from build123d import *
from OCP.BRepFilletAPI import BRepFilletAPI_MakeChamfer

# Parameters (mm, degrees)
BOSS_EXTRUDE1_DEPTH = 3
SKETCH2_R           = 2
CUT_EXTRUDE1_DEPTH  = 31.959580504
CHAMFER1_SIZE       = 2.38
CHAMFER1_SIZE2      = 1.109812226
SKETCH3_R           = 12.7
SKETCH3_R_2         = 11.375
BOSS_EXTRUDE2_DEPTH = 30.75
SKETCH5_W           = 5.58
SKETCH5_H           = 6.85
CUT_EXTRUDE3_DEPTH  = 10
CHAMFER3_SIZE       = 1
CHAMFER3_SIZE2      = 1.191753593
CUT_EXTRUDE4_START  = -5
SKETCH6_R           = 11.375
CUT_EXTRUDE4_DEPTH  = 5
CHAMFER4_SIZE       = 2.4293521
CHAMFER4_SIZE_2     = 3
FILLET1_R           = 0.5
CUT_EXTRUDE6_START  = -35
CUT_EXTRUDE6_DEPTH  = 35


with BuildPart() as part:
    # Sketch1 → Boss-Extrude1 (new body)
    with BuildSketch(Plane.XY):
        with BuildLine():
            Line((6.35, 28.075), (-6.35, 28.075))
            ThreePointArc((-6.35, 28.075), (-10.840128061, 26.215128061), (-12.7, 21.725))
            Line((-12.7, 21.725), (-12.7, -21.725))
            ThreePointArc((-12.7, -21.725), (-10.840128061, -26.215128061), (-6.35, -28.075))
            Line((-6.35, -28.075), (6.35, -28.075))
            ThreePointArc((6.35, -28.075), (10.840128061, -26.215128061), (12.7, -21.725))
            Line((12.7, -21.725), (12.7, 21.725))
            ThreePointArc((12.7, 21.725), (10.840128061, 26.215128061), (6.35, 28.075))
        make_face()
    extrude(amount=BOSS_EXTRUDE1_DEPTH)

    # Sketch2 → Cut-Extrude1 (cut, through all)
    with BuildSketch(Plane(origin=(0, 0, 0), x_dir=(-1, 0, 0), z_dir=(0, 0, -1))):
        with Locations((-7.7, -20.125)):
            Circle(SKETCH2_R)
        with Locations((-7.7, 20.125)):
            Circle(SKETCH2_R)
        with Locations((7.7, 20.125)):
            Circle(SKETCH2_R)
        with Locations((7.7, -20.125)):
            Circle(SKETCH2_R)
    extrude(amount=-CUT_EXTRUDE1_DEPTH, mode=Mode.SUBTRACT)

    # Chamfer1: one chamfer whose edges measure the first distance from different faces: ONE call of the kernel's chamfer builder (chamfer() names one face for all edges)
    chamfer1_edges_1 = [part.edges().sort_by_distance(p)[0] for p in [
        (-10.840128061, 26.215128061, 3),
    ]]
    chamfer1_side_1 = [part.faces().sort_by_distance(p)[0] for p in [
        (-10.840128061, 26.215128061, 1.5),
    ]]
    chamfer1_edges_2 = [part.edges().sort_by_distance(p)[0] for p in [
        (-12.7, 0, 3),
    ]]
    chamfer1_side_2 = [part.faces().sort_by_distance(p)[0] for p in [
        (-12.7, 0, 1.5),
    ]]
    chamfer1_edges_3 = [part.edges().sort_by_distance(p)[0] for p in [
        (-10.840128061, -26.215128061, 3),
    ]]
    chamfer1_side_3 = [part.faces().sort_by_distance(p)[0] for p in [
        (-10.840128061, -26.215128061, 1.5),
    ]]
    chamfer1_edges_4 = [part.edges().sort_by_distance(p)[0] for p in [
        (0, -28.075, 3),
    ]]
    chamfer1_side_4 = [part.faces().sort_by_distance(p)[0] for p in [
        (0, -28.075, 1.5),
    ]]
    chamfer1_edges_5 = [part.edges().sort_by_distance(p)[0] for p in [
        (10.840128061, -26.215128061, 3),
    ]]
    chamfer1_side_5 = [part.faces().sort_by_distance(p)[0] for p in [
        (10.840128061, -26.215128061, 1.5),
    ]]
    chamfer1_edges_6 = [part.edges().sort_by_distance(p)[0] for p in [
        (12.7, 0, 3),
    ]]
    chamfer1_side_6 = [part.faces().sort_by_distance(p)[0] for p in [
        (12.7, 0, 1.5),
    ]]
    chamfer1_edges_7 = [part.edges().sort_by_distance(p)[0] for p in [
        (10.840128061, 26.215128061, 3),
    ]]
    chamfer1_side_7 = [part.faces().sort_by_distance(p)[0] for p in [
        (10.840128061, 26.215128061, 1.5),
    ]]
    chamfer1_edges_8 = [part.edges().sort_by_distance(p)[0] for p in [
        (0, 28.075, 3),
    ]]
    chamfer1_side_8 = [part.faces().sort_by_distance(p)[0] for p in [
        (0, 28.075, 1.5),
    ]]
    chamfer1 = BRepFilletAPI_MakeChamfer(part.part.solid().wrapped)
    for e in chamfer1_edges_1:
        chamfer1.Add(CHAMFER1_SIZE, CHAMFER1_SIZE2, e.wrapped, chamfer1_side_1[0].wrapped)  # the first distance lies on this face
    for e in chamfer1_edges_2:
        chamfer1.Add(CHAMFER1_SIZE, CHAMFER1_SIZE2, e.wrapped, chamfer1_side_2[0].wrapped)  # the first distance lies on this face
    for e in chamfer1_edges_3:
        chamfer1.Add(CHAMFER1_SIZE, CHAMFER1_SIZE2, e.wrapped, chamfer1_side_3[0].wrapped)  # the first distance lies on this face
    for e in chamfer1_edges_4:
        chamfer1.Add(CHAMFER1_SIZE, CHAMFER1_SIZE2, e.wrapped, chamfer1_side_4[0].wrapped)  # the first distance lies on this face
    for e in chamfer1_edges_5:
        chamfer1.Add(CHAMFER1_SIZE, CHAMFER1_SIZE2, e.wrapped, chamfer1_side_5[0].wrapped)  # the first distance lies on this face
    for e in chamfer1_edges_6:
        chamfer1.Add(CHAMFER1_SIZE, CHAMFER1_SIZE2, e.wrapped, chamfer1_side_6[0].wrapped)  # the first distance lies on this face
    for e in chamfer1_edges_7:
        chamfer1.Add(CHAMFER1_SIZE, CHAMFER1_SIZE2, e.wrapped, chamfer1_side_7[0].wrapped)  # the first distance lies on this face
    for e in chamfer1_edges_8:
        chamfer1.Add(CHAMFER1_SIZE, CHAMFER1_SIZE2, e.wrapped, chamfer1_side_8[0].wrapped)  # the first distance lies on this face
    add(Compound.cast(chamfer1.Shape()), mode=Mode.REPLACE)

    # Sketch3 → Boss-Extrude2 (add)
    with BuildSketch(Plane(origin=(0, 0, 0), x_dir=(-1, 0, 0), z_dir=(0, 0, -1))):
        Circle(SKETCH3_R)
        Circle(SKETCH3_R_2, mode=Mode.SUBTRACT)
    extrude(amount=BOSS_EXTRUDE2_DEPTH)

    # Sketch5 → Cut-Extrude3 (cut)
    with BuildSketch(Plane.XY.offset(3)):
        with Locations((-0.000187774, 20.125)):
            Rectangle(SKETCH5_W, SKETCH5_H)
    extrude(amount=-CUT_EXTRUDE3_DEPTH, mode=Mode.SUBTRACT)

    # Chamfer3
    chamfer3_edges = [part.edges().sort_by_distance(p)[0] for p in [
        (2.789812226, 20.125, 0),
        (-0.000187774, 16.7, 0),
        (-2.790187774, 20.125, 0),
        (-0.000187774, 23.55, 0),
    ]]
    chamfer3_side = [part.faces().sort_by_distance(p)[0] for p in [
        (10.572418738, 25.947418738, 0),
    ]]
    chamfer(chamfer3_edges, length=CHAMFER3_SIZE, length2=CHAMFER3_SIZE2, reference=chamfer3_side[0])

    # Sketch6 → Cut-Extrude4 (cut)
    with BuildSketch(Plane(origin=(0, 0, 0), x_dir=(-1, 0, 0), z_dir=(0, 0, -1)).offset(CUT_EXTRUDE4_START)):
        Circle(SKETCH6_R)
    extrude(amount=CUT_EXTRUDE4_DEPTH, mode=Mode.SUBTRACT)

    # Chamfer4
    # the kernel refuses this chamfer: 3, 2.4293521 mm, written as the material it takes off along each edge
    with BuildSketch(Plane(origin=(7.7, -20.125, 3), x_dir=(-1, 0, 0), z_dir=(0, -1, 0))) as chamfer4_piece_1:
        Polygon((2 + CHAMFER4_SIZE, 0), (2, CHAMFER4_SIZE_2), (2, 0), align=None)
    revolve(axis=Axis((7.7, -20.125, 3), (0, 0, -1)), mode=Mode.SUBTRACT)
    with BuildSketch(Plane(origin=(-7.7, 20.125, 3), x_dir=(-1, 0, 0), z_dir=(0, -1, 0))) as chamfer4_piece_2:
        Polygon((2 + CHAMFER4_SIZE, 0), (2, CHAMFER4_SIZE_2), (2, 0), align=None)
    revolve(axis=Axis((-7.7, 20.125, 3), (0, 0, -1)), mode=Mode.SUBTRACT)
    with BuildSketch(Plane(origin=(-7.7, -20.125, 3), x_dir=(-1, 0, 0), z_dir=(0, -1, 0))) as chamfer4_piece_3:
        Polygon((2 + CHAMFER4_SIZE, 0), (2, CHAMFER4_SIZE_2), (2, 0), align=None)
    revolve(axis=Axis((-7.7, -20.125, 3), (0, 0, -1)), mode=Mode.SUBTRACT)
    with BuildSketch(Plane(origin=(7.7, 20.125, 3), x_dir=(-1, 0, 0), z_dir=(0, -1, 0))) as chamfer4_piece_4:
        Polygon((2, CHAMFER4_SIZE_2), (2 + CHAMFER4_SIZE, 0), (2, 0), align=None)
    revolve(axis=Axis((7.7, 20.125, 3), (0, 0, -1)), mode=Mode.SUBTRACT)

    # Fillet1
    # the kernel refuses this fillet: 0.5 mm, written as the material it takes off along each edge
    with BuildSketch(Plane(origin=(0, 0, 3), x_dir=(-1, 0, 0), z_dir=(0, 1, 0))) as fillet1_piece_1:
        with BuildLine():
            CenterArc((11.375 + FILLET1_R, -FILLET1_R), FILLET1_R, 90, 90)
            Line((11.375, -FILLET1_R), (11.375, 0))
            Line((11.375, 0), (11.375 + FILLET1_R, 0))
        make_face()
    revolve(axis=Axis((0, 0, 3), (0, 0, 1)), mode=Mode.SUBTRACT)

    # Sketch7 → Cut-Extrude6 (cut)
    with BuildSketch(Plane(origin=(0, 0, -30.75), x_dir=(-1, 0, 0), z_dir=(0, 0, -1)).offset(CUT_EXTRUDE6_START)):
        with BuildLine():
            Line((-0.85, 11.343197301), (-0.85, 12.75))
            Line((-0.85, 12.75), (0.85, 12.75))
            Line((0.85, 12.75), (0.85, 11.343197301))
            ThreePointArc((0.85, 11.343197301), (0, 11.375), (-0.85, 11.343197301))
        make_face()
    extrude(amount=CUT_EXTRUDE6_DEPTH, mode=Mode.SUBTRACT)


solid = part.part
Here's how the part is built. I have some questions about the finished solid (model axes, mm). A direction names the side the tool comes from. Round coordinates to 2 decimals unless told otherwise and drop trailing zeros. Write each loop counter-clockwise with the first axis right and the second up, starting at its lowest first coordinate (ties: lowest second). Pieces come first, ordered by that corner, then holes.
1. Will these pins go through, and if not, where does the flat tip stop? pin 1 Ø1.4 at (y, z) = (19.5, 2) entering from -X; pin 2 Ø3 at (x, z) = (8.5, -13.5) entering from +Y; pin 3 Ø0.7 at (y, z) = (12, -6) entering from +X; pin 4 Ø6 at (x, y) = (7.5, 3.5) entering from +Z.
2. I need wall thicknesses on L1, parallel to X at y = 0, z = -16 (3 decimals); L2, parallel to Z at x = -9, y = 15; L3, parallel to Y at x = 3, z = -14. Which ranges of each line are inside material? Lowest first, please.
3. Suppose I cut it at C-C (x = -7.7). State how many separate pieces and enclosed holes the cut face has, and give its area (3 significant figures).
4. If we mould it in two halves opening along X, with no side actions, what happens to faces 4 (the conical face through (10.399, 25.686, 2.091)), 5 (the conical face through (-10.311, 25.774, 2.091)), 6 (the flat face through (0, 23.55, 2))? For each: released by +X, released by -X, zero draft, split by the parting line, or undercut.
5. For faces 1 (the flat face through (-0.053, 16.207, 0.604)), 2 (the conical face through (10.311, -25.774, 2.091)), 3 (the flat face through (0, 16.7, 2)), which set-ups out of +Z, -Z, +X, -X, +Y, -Y let a thin tool reach every point of the face, with its end or its side?
6. Suppose I cut it at A-A (x = 0). List the corners of the cut face in (y, z) for me (3 decimals), and give its area (3 significant figures).
7. Suppose I cut it at B-B (z = -4). List the corners of the cut face in (x, y) for me (3 decimals).
Answer sheet:
1. pin 1: stops at x = -12.38
1. pin 2: stops at y = 10.6
1. pin 3: stops at x = 5.06
1. pin 4: passes through
2. L1: x = -12.7 to -11.375, 11.375 to 12.7
2. L2: z = 0 to 3
2. L3: y = -12.34 to -10.97, 10.97 to 12.34
3. separate pieces: 4
3. enclosed holes: 0
3. area: 182 mm2
4. face 4: released by +X
4. face 5: released by -X
4. face 6: undercut
5. face 1: -Z
5. face 2: +Z, +X, -Y
5. face 3: +Z, -Z
6. outline: (-28.075, 0) - (-12.7, 0) - (-12.7, -30.75) - (-11.375, -30.75) - (-11.375, 2.5) arc R0.5 ccw to (-11.875, 3) - (-26.965, 3) - (-28.075, 0.62) - close; (12.75, 0) - (15.7, 0) - (16.7, 1.192) - (16.7, 3) - (12.75, 3) - close; (23.55, 1.192) - (24.55, 0) - (28.075, 0) - (28.075, 0.62) - (26.965, 3) - (23.55, 3) - close
6. area: 112 mm2
7. outline: (-0.85, 11.343) - (-0.85, 12.672) arc R12.7 ccw (long way) to (0.85, 12.672) - (0.85, 11.343) arc R11.375 cw (long way) to start
